```python
from build123d import *

# Parameters (mm, degrees)
F1_DEPTH = 2
F2_DEPTH = 5
F3_DEPTH = 10


with BuildPart() as f1:
    # F0 (on Right) → F1 (new body)
    with BuildSketch(Plane.YZ):
        with BuildLine():
            Line((-33.6863736738, 16.3327330157), (-41.9186067209, 24.5649660628))
            Line((-41.9186067209, 24.5649660628), (-41.9186067209, 4.5649660628))
            Line((-41.9186067209, 4.5649660628), (-33.6863736738, 12.7971991098))
            ThreePointArc((-33.6863736738, 12.7971991098), (-34.4186067209, 14.5649660628), (-33.6863736738, 16.3327330157))
        make_face()
        with BuildLine():
            Line((-21.9186067209, 24.5649660628), (-41.9186067209, 24.5649660628))
            Line((-41.9186067209, 24.5649660628), (-33.6863736738, 16.3327330157))
            ThreePointArc((-33.6863736738, 16.3327330157), (-31.9186067209, 17.0649660628), (-30.1508397679, 16.3327330157))
            Line((-30.1508397679, 16.3327330157), (-21.9186067209, 24.5649660628))
        make_face()
        with BuildLine():
            Line((-21.9186067209, 4.5649660628), (-21.9186067209, 24.5649660628))
            Line((-21.9186067209, 24.5649660628), (-30.1508397679, 16.3327330157))
            ThreePointArc((-30.1508397679, 16.3327330157), (-29.6089078896, 15.5216746437), (-29.4186067209, 14.5649660628))
            ThreePointArc((-29.4186067209, 14.5649660628), (-29.6089078896, 13.6082574819), (-30.1508397679, 12.7971991098))
            Line((-30.1508397679, 12.7971991098), (-21.9186067209, 4.5649660628))
        make_face()
        with BuildLine():
            Line((-33.6863736738, 12.7971991098), (-41.9186067209, 4.5649660628))
            Line((-41.9186067209, 4.5649660628), (-21.9186067209, 4.5649660628))
            Line((-21.9186067209, 4.5649660628), (-30.1508397679, 12.7971991098))
            ThreePointArc((-30.1508397679, 12.7971991098), (-31.9186067209, 12.0649660628), (-33.6863736738, 12.7971991098))
        make_face()
        with BuildLine():
            Line((-31.9186067209, 14.5649660628), (-33.6863736738, 16.3327330157))
            ThreePointArc((-33.6863736738, 16.3327330157), (-34.4186067209, 14.5649660628), (-33.6863736738, 12.7971991098))
            Line((-33.6863736738, 12.7971991098), (-31.9186067209, 14.5649660628))
        make_face()
        with BuildLine():
            ThreePointArc((-30.1508397679, 16.3327330157), (-31.9186067209, 17.0649660628), (-33.6863736738, 16.3327330157))
            Line((-33.6863736738, 16.3327330157), (-31.9186067209, 14.5649660628))
            Line((-31.9186067209, 14.5649660628), (-30.1508397679, 16.3327330157))
        make_face()
        with BuildLine():
            ThreePointArc((-29.4186067209, 14.5649660628), (-29.6089078896, 15.5216746437), (-30.1508397679, 16.3327330157))
            Line((-30.1508397679, 16.3327330157), (-31.9186067209, 14.5649660628))
            Line((-31.9186067209, 14.5649660628), (-30.1508397679, 12.7971991098))
            ThreePointArc((-30.1508397679, 12.7971991098), (-29.6089078896, 13.6082574819), (-29.4186067209, 14.5649660628))
        make_face()
        with BuildLine():
            Line((-31.9186067209, 14.5649660628), (-33.6863736738, 12.7971991098))
            ThreePointArc((-33.6863736738, 12.7971991098), (-31.9186067209, 12.0649660628), (-30.1508397679, 12.7971991098))
            Line((-30.1508397679, 12.7971991098), (-31.9186067209, 14.5649660628))
        make_face()
    extrude(amount=F1_DEPTH)

    # F0 (on Right) → F2 (join)
    with BuildSketch(Plane.YZ):
        with BuildLine():
            ThreePointArc((-29.4186067209, 14.5649660628), (-29.6089078896, 15.5216746437), (-30.1508397679, 16.3327330157))
            Line((-30.1508397679, 16.3327330157), (-31.9186067209, 14.5649660628))
            Line((-31.9186067209, 14.5649660628), (-30.1508397679, 12.7971991098))
            ThreePointArc((-30.1508397679, 12.7971991098), (-29.6089078896, 13.6082574819), (-29.4186067209, 14.5649660628))
        make_face()
        with BuildLine():
            ThreePointArc((-30.1508397679, 16.3327330157), (-31.9186067209, 17.0649660628), (-33.6863736738, 16.3327330157))
            Line((-33.6863736738, 16.3327330157), (-31.9186067209, 14.5649660628))
            Line((-31.9186067209, 14.5649660628), (-30.1508397679, 16.3327330157))
        make_face()
        with BuildLine():
            Line((-31.9186067209, 14.5649660628), (-33.6863736738, 16.3327330157))
            ThreePointArc((-33.6863736738, 16.3327330157), (-34.4186067209, 14.5649660628), (-33.6863736738, 12.7971991098))
            Line((-33.6863736738, 12.7971991098), (-31.9186067209, 14.5649660628))
        make_face()
        with BuildLine():
            Line((-31.9186067209, 14.5649660628), (-33.6863736738, 12.7971991098))
            ThreePointArc((-33.6863736738, 12.7971991098), (-31.9186067209, 12.0649660628), (-30.1508397679, 12.7971991098))
            Line((-30.1508397679, 12.7971991098), (-31.9186067209, 14.5649660628))
        make_face()
    extrude(amount=-F2_DEPTH)

    # F3 (add): a face of the model
    f3_faces = [f1.faces().sort_by_distance(p)[0] for p in [
        (1, -31.9186067209, 24.5649660628),
    ]]
    extrude(f3_faces, amount=F3_DEPTH)


solid = f1.part
```
Can you work these out from the model? Positions are in its coordinate system, mm. Coordinates: 2 decimals unless noted, no trailing zeros. Loops run counter-clockwise (first coordinate to the right, second up) from the corner with the lowest first, then second, coordinate; pieces in that order, holes last.
1) Imagine slicing it at B-B on y = -33. List the corners of the cut face in (x, z) for me.
2) Imagine slicing it at C-C on z = 12.5. List the corners of the cut face in (x, y) for me.
3) I need wall thicknesses on probe 1 along X at (y, z) = (-34.5, 12); probe 2 along Y at (x, z) = (-1, 14.5); probe 3 along Y at (x, z) = (-3, 14). Which ranges of each line are inside material? Lowest first, please.
4) Imagine slicing it at D-D on y = -39.5. List the corners of the cut face in (x, z) for me, plus the area to 3 significant figures.
5) Imagine slicing it at A-A on x = -1. List the corners of the cut face in (y, z) for me.
6) For pin 1 (12 mm diameter, centred on y = -29.5, z = 22, fed in from -X); pin 2 (1 mm diameter, centred on x = -1.5, z = 15, fed in from +Y), each with a flat end and sliding along its axis, tell me the tip position at first contact or that it passes through.
Completed:
1. outline: (-5, 12.31) - (0, 12.31) - (0, 4.56) - (2, 4.56) - (2, 34.56) - (0, 34.56) - (0, 16.82) - (-5, 16.82) - close
2. outline: (-5, -33.33) - (0, -33.33) - (0, -41.92) - (2, -41.92) - (2, -21.92) - (0, -21.92) - (0, -30.51) - (-5, -30.51) - close
3. probe 1: x = 0 to 2
3. probe 2: y = -34.42 to -29.42
3. probe 3: y = -34.35 to -29.48
4. outline: (0, 4.56) - (2, 4.56) - (2, 34.56) - (0, 34.56) - close
4. area: 60.0 mm2
5. outline: circle Ø5 at (-31.92, 14.56)
6. pin 1: stops at x = -5
6. pin 2: stops at y = -29.42
